```python
from build123d import *

# Parameters (mm, degrees)
SKETCH1_R           = 9.525
BOSS_EXTRUDE1_DEPTH = 3.175
CHAMFER1_SIZE       = 0.06
CHAMFER2_SIZE       = 0.06


with BuildPart() as part:
    # Sketch1 → Boss-Extrude1 (new body)
    with BuildSketch(Plane(origin=(0, 0, 0), x_dir=(1, 0, 0), z_dir=(0, 1, 0))):
        with Locations(Location((0, 0, 0), (0, 0, 270))):
            Circle(SKETCH1_R)
        Polygon((0, 7.216878365), (-6.25, 3.608439182), (-6.25, -3.608439182), (0, -7.216878365), (6.25, -3.608439182), (6.25, 3.608439182), align=None, mode=Mode.SUBTRACT)
    extrude(amount=BOSS_EXTRUDE1_DEPTH)

    # Chamfer1
    chamfer1_edges = [part.edges().sort_by_distance(p)[0] for p in [
        (0, 0, -9.525),
    ]]
    chamfer(chamfer1_edges, length=CHAMFER1_SIZE)

    # Chamfer2
    chamfer2_edges = [part.edges().sort_by_distance(p)[0] for p in [
        (0, 3.175, -9.525),
    ]]
    chamfer(chamfer2_edges, length=CHAMFER2_SIZE)


solid = part.part
```
Input: part model. Units: mm. Frame: model coordinates. A direction names the side the tool comes from. Give positions to 0.01 mm unless a question says otherwise; leave off trailing zeros. Order: outer loops, then holes, each group sorted by start corner. A loop starts at its lowest first (then second) coordinate and runs counter-clockwise, first axis right, second up.
1. Cut plane A-A (z = 0). Return loops of the section in (x, y) (3 decimals), and give its area (3 significant figures).
Computed:
outline: (-9.525, 0.06) - (-9.465, 0) - (-6.25, 0) - (-6.25, 3.175) - (-9.465, 3.175) - (-9.525, 3.115) - close; (6.25, 0) - (9.465, 0) - (9.525, 0.06) - (9.525, 3.115) - (9.465, 3.175) - (6.25, 3.175) - close
area: 20.8 mm2
2. Draft query along Z for faces 3 (the face through (2.2, 3.175, 6.2)), 4 (the face through (-6.25, 2, 0)), 5 (the face through (-5.796, 1.566, -7.559)). Return one class per face: released by +Z, released by -Z, zero draft, split by the parting line, or undercut.
Computed:
face 3: zero draft
face 4: undercut
face 5: split by the parting line
3. Set-up query: faces 1 (the face through (2.2, 0, 6.2)), 2 (the face through (3.08, 1.57, 5.44)). Return all of +Z, -Z, +X, -X, +Y, -Y with unobstructed straight access to the full face (end or side cutting, diameter ignored); none if empty.
Computed:
face 1: +Z, -Z, +X, -X, -Y
face 2: +Y, -Y
4. Cut plane B-B (y = 1.35). Return loops of the section in (x, z) (3 decimals), and give its area (3 significant figures).
Computed:
outline: circle Ø19.05 at (0, 0); hole (-6.25, -3.608) - (0, -7.217) - (6.25, -3.608) - (6.25, 3.608) - (0, 7.217) - (-6.25, 3.608) - close
area: 150 mm2
5. Pin query (flat end, axial travel): pin 1 Ø1.6 at (y, z) = (1, -1) entering from +X. Return the tip coordinate at first contact, or that it passes through.
Computed:
pin 1: stops at x = 9.52
6. Line query: probe 1 along Z at (x, y) = (-1, 1.45); probe 2 along Z at (x, y) = (4, 1.25); probe 3 along X at (y, z) = (2.4, -2). Output: solid intervals per line, ascending.
Computed:
probe 1: z = -9.47 to -6.64, 6.64 to 9.47
probe 2: z = -8.64 to -4.91, 4.91 to 8.64
probe 3: x = -9.31 to -6.25, 6.25 to 9.31
